Autodesk Inventor part; units mm, degrees
ref_plane "YZ Plane" through (0, 0, 0) normal (1, 0, 0) x (0, 1, 0)
ref_plane "XZ Plane" through (0, 0, 0) normal (0, 1, 0) x (-1, 0, 0)
ref_plane "XY Plane" through (0, 0, 0) normal (0, 0, 1) x (1, 0, 0)
sketch "Sketch1" plane through (0, 0, 0) normal (0, 0, 1) x (1, 0, 0)
  line L0 (-26.0293, 0) -> (0, 0)
  line L1 (0, 0) -> (26.0293, 0)
  line L2 (0, 0) -> (0, 50) construction
  line L3 (0, 50) -> (29, 50)
  line L4 (29, 50) -> (29, 47.5)
  line L5 (29, 47.5) -> (5, 43.5)
  line L6 (5, 43.5) -> (5, 22.5)
  line L7 (5, 22.5) -> (29, 16)
  line L8 (29, 16) -> (29, 12.5)
  line L9 (29, 12.5) -> (0, 12.5)
  line L10 (0, 50) -> (-29, 50)
  line L11 (-29, 47.5) -> (-5, 43.5)
  line L12 (-5, 43.5) -> (-5, 22.5)
  line L13 (-5, 22.5) -> (-29, 16)
  line L14 (-29, 16) -> (-29, 12.5)
  line L15 (-29, 12.5) -> (0, 12.5)
  line L16 (-29, 50) -> (-29, 47.5)
  point P0 (14.5, 12.5)
  point P1 (-14.5, 12.5)
  point P2 (-5, 33)
  dimension "d0" = 100
  dimension "d1" = 95
  dimension "d2" = 87
  dimension "d3" = 45
  dimension "d4" = 25
  dimension "d5" = 32
  dimension "d6" = 58
  dimension "d7" = 10
revolve "Revolution1" add sketch "Sketch1" angle 360 about axis through (-26.0293, 0, 0) along (1, 0, 0)
fillet "Fillet1" radius 6 4 edges at (5, -43.5, 0) (5, -22.5, 0) (-5, -43.5, 0) (-5, -22.5, 0)
properties part number "04-roller" material "Stainless Steel"
Can you work these out from the model? Positions are in its coordinate system, mm. A direction names the side the tool comes from. Coordinates: 2 decimals unless noted, no trailing zeros. Write each loop counter-clockwise with the first axis right and the second up, starting at its lowest first coordinate (ties: lowest second). Pieces come first, ordered by that corner, then holes. Notation, with made-up numbers: (27.25, 37) -> (39.25, 37) arc R7 ccw to (39.25, 44) -> close; hole circle Ø1 at (26.25, -37.75). An arc over 180 degrees is marked (long way). Write each question's results on one line, items separated by ' | '. Start each with the question number.
Item 1: Please list where these lines run through material, in increasing order: probe 1 along Z at (x, y) = (2, 0); probe 2 along Z at (x, y) = (8.5, 14.5); probe 3 along Z at (x, y) = (10.5, 0).
Item 2: On a 3-axis mill with a long thin cutter (end or side, diameter ignored), from which of +Z, -Z, +X, -X, +Y, -Y can I reach the whole of each face in a straight line? I mean faces 1 (the flat face through (-29, 44.2, -18.3)), 2 (the flat face through (-5, -26.1, -8)), 3 (the flat face through (5, -26.1, -8)). Say none if no direction works.
Item 3: If we section it at D-D, the plane x = -3.5: Write out the boundary of the cut face in (y, z).
Item 4: Thinking about a two-plate mould opening in Z: for faces 4 (the flat face through (-29, -10, -8)), 5 (the cylindrical face through (0.41, 47.69, 15.02)), 6 (the conical face through (23.43, -2.28, -17.36)), which applies, released by +Z, released by -Z, zero draft, split by the parting line, or undercut?
Item 5: I'm going to push flat-ended pins straight in: P1, Ø8, axis at y = -23, z = 15, coming from the -X side; P2, Ø10, axis at x = 16.5, z = 14, coming from the -Y side; P3, Ø15, axis at y = 0, z = 0, coming from the +X side; P4, Ø4, axis at x = 16, z = -32.5, coming from the -Y side. Where does each tip first touch, or does it pass through?
Item 6: If we section it at C-C, the plane x = -14: Write out the boundary of the cut face in (y, z) (1 decimal), and give its area (3 significant figures).
Answer block:
1) probe 1: -50 to -12.5, 12.5 to 50 | probe 2: -47.85 to -41.41, -16.06 to 16.06, 41.41 to 47.85 | probe 3: -50 to -44.42, -21.01 to -12.5, 12.5 to 21.01, 44.42 to 50
2) face 1: +Z, -Z, -X, +Y, -Y | face 2: -X | face 3: +X
3) outline: circle Ø100 at (0, 0); hole circle Ø25 at (0, 0)
4) face 4: zero draft | face 5: split by the parting line | face 6: undercut
5) P1: x = -6.22 | P2: y = -49.18 | P3: through | P4: y = -39.62
6) outline: circle Ø100 at (0, 0); circle Ø40.1 at (0, 0); hole circle Ø90 at (0, 0); hole circle Ø25 at (0, 0) | area: 2,270 mm²
